Could you check a few things on this model? Use its own coordinates, in mm. Face numbers are marked on the shaded views. A direction names the side the tool comes from. Give positions to 0.01 mm unless a question says otherwise; leave off trailing zeros. Order: outer loops, then holes, each group sorted by start corner. A loop starts at its lowest first (then second) coordinate and runs counter-clockwise, first axis right, second up.
(1) Imagine slicing it at A-A, the plane z = 293.5. Write out the boundary of the cut face in (x, y).
(2) Imagine slicing it at D-D, the plane y = -15. Write out the boundary of the cut face in (x, z), then the cut area to 3 significant figures.
(3) If we mould it in two halves opening along Y, with no side actions, what happens to the marked faces 3, 4 and 5? For each: released by +Y, released by -Y, zero draft, split by the parting line, or undercut.
(4) On a 3-axis mill with a long thin cutter (end or side, diameter ignored), from which of +Z, -Z, +X, -X, +Y, -Y can I reach the whole of each face in a straight line? I mean the marked faces 1 and 2. Say none if no direction works.
(5) Imagine slicing it at C-C, the plane z = 149. Write out the boundary of the cut face in (x, y), then the cut area to 3 significant figures.
(6) If I drill on probe 1 along X at (y, z) = (70, 60.5); probe 2 along Y at (x, z) = (120.5, 50.5); probe 3 along Z at (x, y) = (192.5, -34.5), over which ranges is the centre line in solid material (lowest first)?
(7) Imagine slicing it at B-B, the plane x = 189. Write out the boundary of the cut face in (y, z).
(8) Will this pin go through, and if not, where does the flat tip stop? pin 1 (1 mm diameter, centred on x = 192, y = -52.5, fed in from +Z).
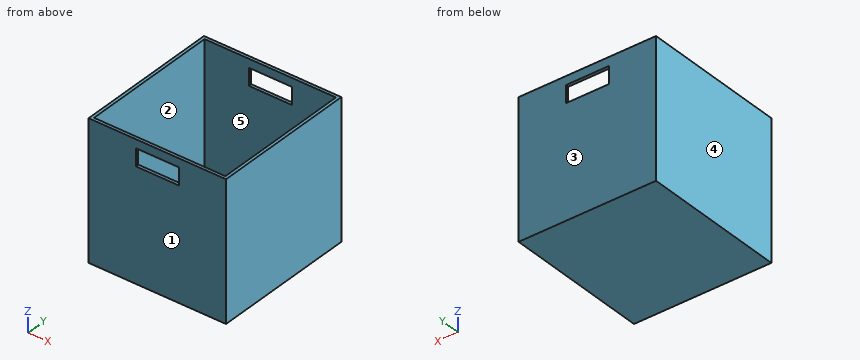
from build123d import *

# Parameters (mm, degrees)
F0_W     = 320
F0_H     = 320
F1_DEPTH = 170
F2_T     = -7
F3_W     = 100
F3_H     = 40
F4_DEPTH = 340.001


with BuildPart() as f1:
    # F0 (on Front) → F1 (new body, symmetric)
    with BuildSketch(Plane.XZ):
        with Locations((160, 160)):
            Rectangle(F0_W, F0_H)
    extrude(amount=F1_DEPTH, both=True)

    # F2
    f2_openings = [f1.faces().sort_by_distance(p)[0] for p in [
        (160, 0, 320),
    ]]
    offset(amount=F2_T, openings=f2_openings)

    # F3 (on face) → F4 (cut, through all)
    with BuildSketch(Plane.XZ.offset(170)):
        with Locations((160, 280)):
            Rectangle(F3_W, F3_H)
    extrude(amount=-F4_DEPTH, mode=Mode.SUBTRACT)


solid = f1.part
Answer block:
1. outline: (0, -170) - (110, -170) - (110, -163) - (7, -163) - (7, 163) - (110, 163) - (110, 170) - (0, 170) - close; (210, -170) - (320, -170) - (320, 170) - (210, 170) - (210, 163) - (313, 163) - (313, -163) - (210, -163) - close
2. outline: (0, 0) - (320, 0) - (320, 320) - (313, 320) - (313, 7) - (7, 7) - (7, 320) - (0, 320) - close
2. area: 6,620 mm2
3. face 3: released by +Y
3. face 4: zero draft
3. face 5: undercut
4. face 1: +Z, -Z, +X, -X, -Y
4. face 2: +Z
5. outline: (0, -170) - (320, -170) - (320, 170) - (0, 170) - close; hole (7, -163) - (313, -163) - (313, 163) - (7, 163) - close
5. area: 9,040 mm2
6. probe 1: x = 0 to 7, 313 to 320
6. probe 2: y = -170 to -163, 163 to 170
6. probe 3: z = 0 to 7
7. outline: (-170, 0) - (170, 0) - (170, 260) - (163, 260) - (163, 7) - (-163, 7) - (-163, 260) - (-170, 260) - close; (-170, 300) - (-163, 300) - (-163, 320) - (-170, 320) - close; (163, 300) - (170, 300) - (170, 320) - (163, 320) - close
8. pin 1: stops at z = 7
